Could you check a few things on this drawing? It's one solid part, dimensions in mm from its lowest x, y, z. A direction names the side the tool comes from. Give positions to 0.01 mm unless a question says otherwise; leave off trailing zeros. Order: outer loops, then holes, each group sorted by start corner. A loop starts at its lowest first (then second) coordinate and runs counter-clockwise, first axis right, second up.
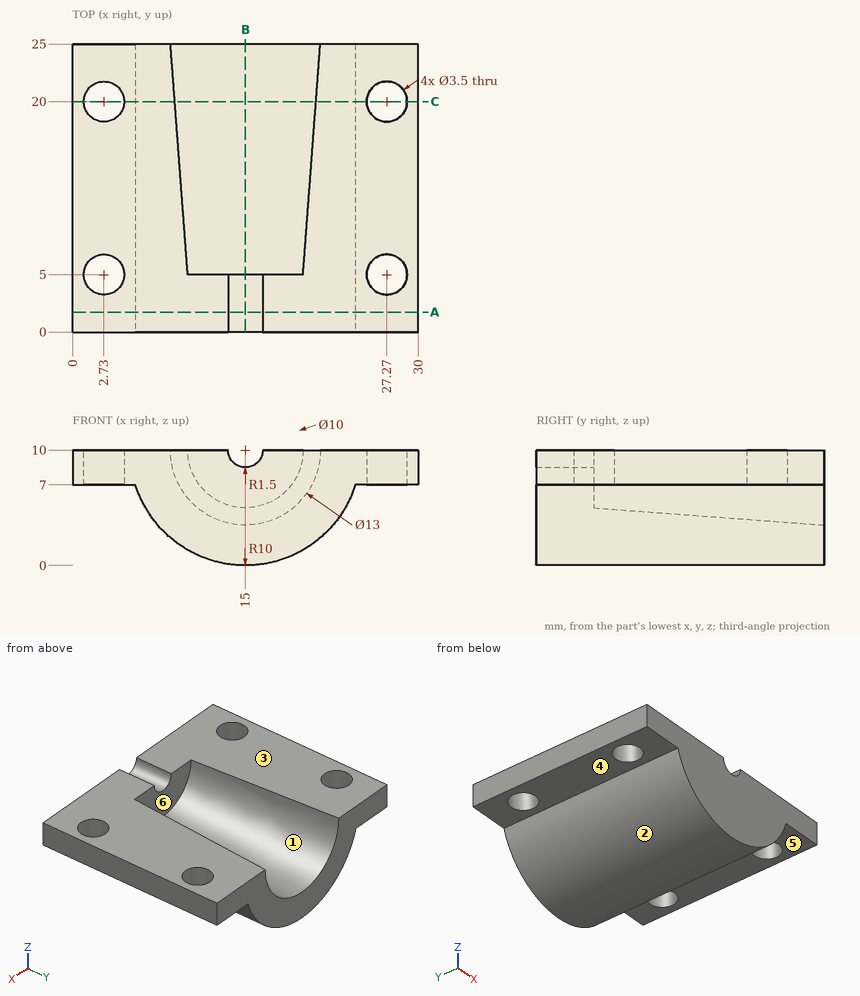
Item 1: We'd pull the mould along X, two halves only. Please class the marked faces 1, 2 and 3: +X half, -X half, draft (parallel to the pull), parting line (faces both ways), or undercut.
Findings:
face 1: undercut
face 2: parting line
face 3: draft
Item 2: For pin 1 (2.5 mm diameter, centred on x = 4, y = 7.5, fed in from -Z); pin 2 (2 mm diameter, centred on y = 6.5, z = 1.5, fed in from -X) (1 decimal); pin 3 (1.5 mm diameter, centred on x = 3.5, y = 5.5, fed in from -Z); pin 4 (1.5 mm diameter, centred on x = 8.5, z = 7, fed in from -Y), each with a flat end and sliding along its axis, tell me the tip position at first contact or that it passes through.
Findings:
pin 1: stops at z = 7
pin 2: stops at x = 8.4
pin 3: passes through
pin 4: stops at y = 0
Item 3: Imagine slicing it at B-B on x = 15. List the corners of the cut face in (y, z) for me.
Findings:
outline: (0, 0) - (25, 0) - (25, 3.5) - (5, 5) - (5, 8.5) - (0, 8.5) - close
Item 4: Please list where these lines run through material, in increasing order: line 1 along Z through (x, y) = (26, 12.75); line 2 along X through (y, z) = (20.75, 5.5); line 3 along Y through (x, z) = (16.5, 8.5).
Findings:
line 1: z = 7 to 10
line 2: x = 6.07 to 10.76, 19.24 to 23.93
line 3: y = 0 to 5
Item 5: Imagine slicing it at A-A on y = 1.75. List the corners of the cut face in (x, z) for me.
Findings:
outline: (0, 7) - (5.46, 7) arc R10 ccw to (24.54, 7) - (30, 7) - (30, 10) - (16.5, 10) arc R1.5 cw to (13.5, 10) - (0, 10) - close
Item 6: For the marked faces 4, 5 and 6, which set-ups out of +Z, -Z, +X, -X, +Y, -Y let a thin tool reach every point of the face, with its end or its side?
Findings:
face 4: -Z, -X, +Y, -Y
face 5: -Z, +X, +Y, -Y
face 6: +Z, +Y
Item 7: Imagine slicing it at C-C on y = 20. Give the number of separate pieces and of enclosed holes in the cut face, then the cut area to 3 significant figures.
Findings:
separate pieces: 3
enclosed holes: 0
area: 108 mm2
